Geometry: see drawing. Coordinates: mm, zero at the bounding-box minimum. Give positions to 0.01 mm unless a question says otherwise; leave off trailing zeros. Loops run counter-clockwise (first coordinate to the right, second up) from the corner with the lowest first, then second, coordinate; pieces in that order, holes last. Notation, with made-up numbers: M 43,13 L 75,13 A20 ccw 75,28 Z; hole C 19.25,6.5 d10. An arc over 180 degrees is marked long. Answer in a Markdown table with one row per item.
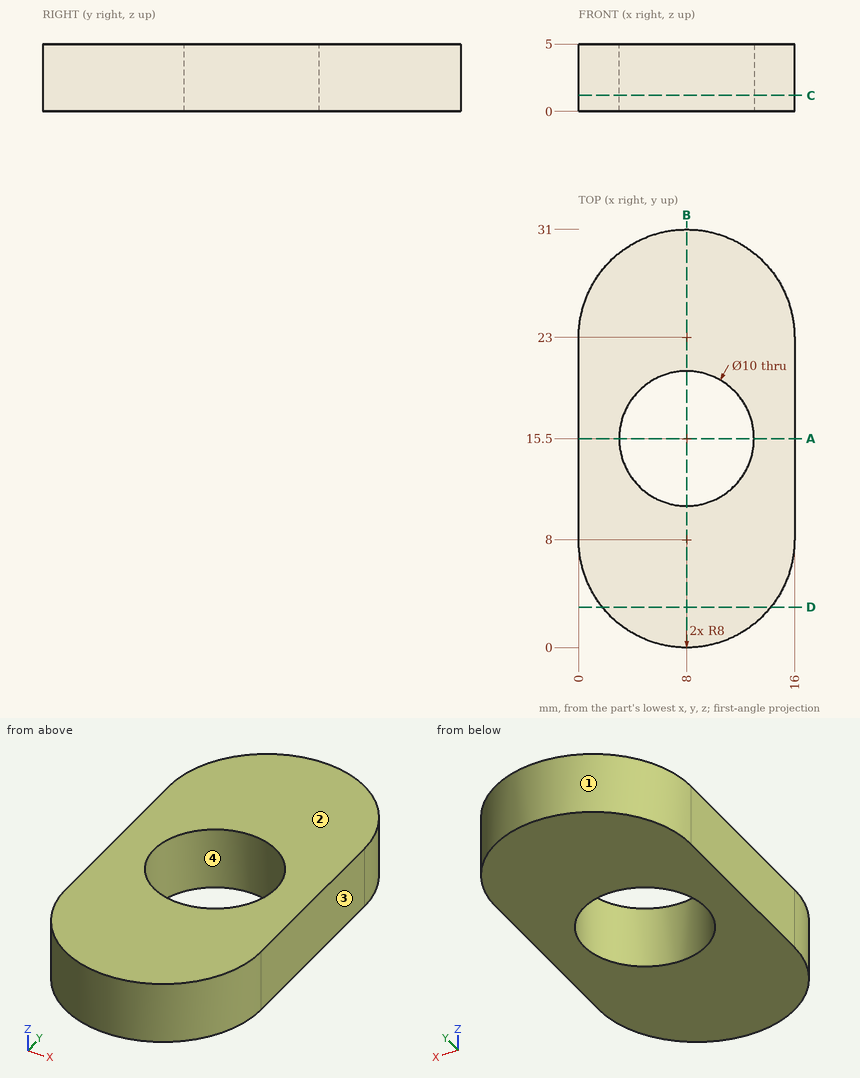
1) Section D-D, the plane y = 3. Return loops of the section in (x, z) (3 decimals), then the cut area to 4 significant figures.
Reply:
| item | result |
|---|---|
| outline | M 1.755,0 L 14.245,0 L 14.245,5 L 1.755,5 Z |
| area | 62.45 mm² |
2) Material intervals for L1, parallel to Y at x = 8, z = 3.7; L2, parallel to X at y = 18, z = 1.6; L3, parallel to X at y = 16.5, z = 3.4, sorted ascending.
Reply:
| item | result |
|---|---|
| L1 | y = 0 to 10.5, 20.5 to 31 |
| L2 | x = 0 to 3.67, 12.33 to 16 |
| L3 | x = 0 to 3.1, 12.9 to 16 |
3) Pin query (flat end, axial travel): pin 1 Ø2 at (x, z) = (4, 3.5) entering from -Y. Return the tip coordinate at first contact, or that it passes through.
Reply:
| item | result |
|---|---|
| pin 1 | stops at y = 0.58 |
4) Pull-direction query (X, two-part tool) for the marked faces 1, 2, 3 and 4; classes: released by +X, released by -X, zero draft, split by the parting line, or undercut.
Reply:
| item | result |
|---|---|
| face 1 | split by the parting line |
| face 2 | zero draft |
| face 3 | released by +X |
| face 4 | undercut |
5) Section B-B, the plane x = 8. Return loops of the section in (y, z), then the cut area to 3 significant figures.
Reply:
| item | result |
|---|---|
| outline | M 0,0 L 10.5,0 L 10.5,5 L 0,5 Z; M 20.5,0 L 31,0 L 31,5 L 20.5,5 Z |
| area | 105 mm² |
6) Section C-C, the plane z = 1.2. Return loops of the section in (x, y), then the cut area to 3 significant figures.
Reply:
| item | result |
|---|---|
| outline | M 0,8 A8 ccw 16,8 L 16,23 A8 ccw 0,23 Z; hole C 8,15.5 d10 |
| area | 363 mm² |
7) Section A-A, the plane y = 15.5. Return loops of the section in (x, z).
Reply:
| item | result |
|---|---|
| outline | M 0,0 L 3,0 L 3,5 L 0,5 Z; M 13,0 L 16,0 L 16,5 L 13,5 Z |
